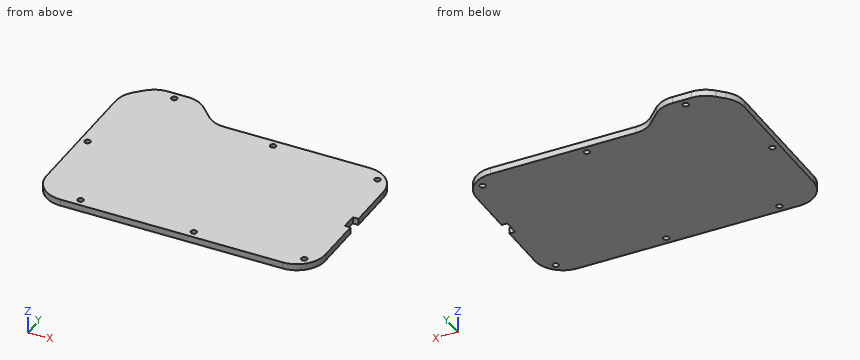
from build123d import *

# Parameters (mm, degrees)
SKETCH1_R           = 1.425
BOSS_EXTRUDE1_DEPTH = 3.175


with BuildPart() as part:
    # Sketch1 → Boss-Extrude1 (new body)
    with BuildSketch(Plane.XY):
        with BuildLine():
            Line((143.808069079, 20.460501739), (143.808069079, 44.360501739))
            Line((143.808069079, 44.360501739), (141.058069079, 44.360501739))
            Line((141.058069079, 44.360501739), (141.058069079, 51.860501739))
            Line((141.058069079, 51.860501739), (143.808069079, 51.860501739))
            Line((143.808069079, 51.860501739), (143.808069079, 75.76050174))
            ThreePointArc((143.808069079, 75.76050174), (139.780787321, 85.483219981), (130.058069079, 89.51050174))
            Line((130.058069079, 89.51050174), (59.375183039, 89.51050174))
            ThreePointArc((59.375183039, 89.51050174), (54.476835105, 90.484843724), (50.32421624, 93.259534941))
            Line((50.32421624, 93.259534941), (44.500531199, 99.083219981))
            ThreePointArc((44.500531199, 99.083219981), (40.039710153, 102.063845312), (34.777812958, 103.11050174))
            Line((34.777812958, 103.11050174), (25.414810921, 103.11050174))
            ThreePointArc((25.414810921, 103.11050174), (20.152913726, 102.063845312), (15.69209268, 99.083219981))
            Line((15.69209268, 99.083219981), (12.411836559, 95.80296386))
            ThreePointArc((12.411836559, 95.80296386), (9.431211228, 91.342142814), (8.3845548, 86.080245619))
            Line((8.3845548, 86.080245619), (8.3845548, 20.460501739))
            ThreePointArc((8.3845548, 20.460501739), (12.411836559, 10.737783497), (22.1345548, 6.710501739))
            Line((22.1345548, 6.710501739), (130.058069079, 6.710501739))
            ThreePointArc((130.058069079, 6.710501739), (139.780787321, 10.737783497), (143.808069079, 20.460501739))
        make_face()
        with Locations((12.0345548, 52.470373679)):
            Circle(SKETCH1_R, mode=Mode.SUBTRACT)
        with Locations((30.09631194, 99.46050174)):
            Circle(SKETCH1_R, mode=Mode.SUBTRACT)
        with Locations((85.053742799, 85.86050174)):
            Circle(SKETCH1_R, mode=Mode.SUBTRACT)
        with Locations((137.199847569, 82.902280229)):
            Circle(SKETCH1_R, mode=Mode.SUBTRACT)
        with Locations((137.199847569, 13.318723249)):
            Circle(SKETCH1_R, mode=Mode.SUBTRACT)
        with Locations((85.053742799, 10.36050174)):
            Circle(SKETCH1_R, mode=Mode.SUBTRACT)
        with Locations((30.09631194, 10.36050174)):
            Circle(SKETCH1_R, mode=Mode.SUBTRACT)
    extrude(amount=BOSS_EXTRUDE1_DEPTH)


solid = part.part
Can you work these out from the model? Positions are in its coordinate system, mm. Round coordinates to 2 decimals unless told otherwise and drop trailing zeros. Write each loop counter-clockwise with the first axis right and the second up, starting at its lowest first coordinate (ties: lowest second). Pieces come first, ordered by that corner, then holes. Notation, with made-up numbers: M 88,57 L 127,57 A29 cw 127,93 Z; hole C -27.5,-13.5 d9. An arc over 180 degrees is marked long. Use a Markdown table: item, result.
Item 1: I want a section at B-B (x = 126). List the corners of the cut face in (y, z) for me (1 decimal).
Found:
| item | result |
|---|---|
| outline | M 6.7,0 L 89.5,0 L 89.5,3.2 L 6.7,3.2 Z |
Item 2: If I drill on line 1 along Y through (x, z) = (30, 0.15); line 2 along Y through (x, z) = (86, 0.7); line 3 along Y through (x, z) = (66, 3), over which ranges is the centre line in solid material (lowest first)? Write a range as [from, to].
Found:
| item | result |
|---|---|
| line 1 | y = [6.71, 8.94], [11.78, 98.04], [100.88, 103.11] |
| line 2 | y = [6.71, 9.3], [11.43, 84.8], [86.93, 89.51] |
| line 3 | y = [6.71, 89.51] |
Item 3: I want a section at A-A (z = 2.65). State how many separate pieces and enclosed holes the cut face has, and give its area (3 significant figures).
Found:
| item | result |
|---|---|
| separate pieces | 1 |
| enclosed holes | 7 |
| area | 11,500 mm2 |
Item 4: For pin 1 Ø3.5 at (x, y) = (137.2, 82.9) entering from -Z; pin 2 Ø1.6 at (y, z) = (47, 2) entering from +X; pin 3 Ø1 at (x, z) = (81, 2) entering from +Y, each with a flat end and sliding along its axis, tell me the tip position at first contact or that it passes through.
Found:
| item | result |
|---|---|
| pin 1 | stops at z = 0 |
| pin 2 | stops at x = 141.06 |
| pin 3 | stops at y = 89.51 |
